```python
from build123d import *

# Parameters (mm, degrees)
BOSS_EXTRUDE1_DEPTH = 5
SKETCH2_R           = 2.55
CUT_EXTRUDE1_DEPTH  = 131.560330882
FILLET1_R           = 5


with BuildPart() as part:
    # Sketch1 → Boss-Extrude1 (new, symmetric)
    with BuildSketch(Plane.XY):
        Polygon((-49.7, 1.55), (-49.7, -11), (-5.15, -11), (-5.15, 0), (5.15, 0), (5.15, -11), (49.7, -11), (49.7, 1.55), (56, 1.55), (65, 1.55), (65, 8.55), (-65, 8.55), (-65, 1.55), (-56, 1.55), align=None)
    extrude(amount=BOSS_EXTRUDE1_DEPTH, both=True)

    # Sketch2 → Cut-Extrude1 (cut, through all)
    with BuildSketch(Plane.ZY.offset(65)):
        with Locations((0, -5.95)):
            Circle(SKETCH2_R)
    extrude(amount=-CUT_EXTRUDE1_DEPTH, mode=Mode.SUBTRACT)

    # Fillet1
    fillet1_edges = [part.edges().sort_by_distance(p)[0] for p in [
        (-27.425, -11, 5),
        (27.425, -11, 5),
        (-27.425, -11, -5),
        (27.425, -11, -5),
    ]]
    fillet(fillet1_edges, radius=FILLET1_R - 0.0001)  # a hair under: the kernel refuses the full size


solid = part.part
```
The listing builds one solid part. Answer for the finished solid, in the listing's coordinates (mm). A direction names the side the tool comes from. Coordinates: 2 decimals unless noted, no trailing zeros. Loops run counter-clockwise (first coordinate to the right, second up) from the corner with the lowest first, then second, coordinate; pieces in that order, holes last. Notation, with made-up numbers: M 8.5,-9 L 49.5,-9 A23 ccw 49.5,18 Z; hole C 19,84.5 d10. An arc over 180 degrees is marked long. Answer as a JSON object with one key per item and string values. Group by question number.
Item 1: Which of the six approach directions +Z, -Z, +X, -X, +Y, -Y give full straight-line access (tool end or side, diameter ignored) to faces 1 (the face through (-49.7, -3, 0)), 2 (the face through (57, 1.55, 0)), 3 (the face through (-5.15, -3, 0)), 4 (the face through (27.1, -8.2, 1.2)), 5 (the face through (-65, 5, 0))?
Item 2: Section A-A (y = -2) is taken. Write down the section's boundary in (x, z).
Item 3: Determine the mould class of faces 6 (the face through (0, 0, 0)), 7 (the face through (-1, 1, 5)), 8 (the face through (5.15, -3, 0)), 9 (the face through (49.7, -3, 1)) for opening direction X: +X half, -X half, draft (parallel to the pull), parting line (faces both ways), or undercut.
Item 4: Each of these flat-tipped pins is pushed along its axis until it touches: P1, Ø3, axis at x = 2, z = 0.5, coming from the -Y side; P2, Ø3, axis at y = -3, z = 2, coming from the -X side; P3, Ø3, axis at y = -6, z = 1.5, coming from the +X side. Where does it stop, or does it pass through?
Item 5: Consider L1, parallel to X at y = -3.25, z = -3; L2, parallel to Y at x = -30.5, z = 0; L3, parallel to X at y = 1, z = -4.5. Determine where each line is inside the solid, lowest interval first.
Item 6: Section C-C (x = -1.5) is taken. Write down the section's boundary in (y, z).
Solved:
{
 "1": {"face 1": "+Z, -Z, -X, -Y", "face 2": "+Z, -Z, +X, -Y", "face 3": "+Z, -Z, -Y", "face 4": "+X, -X", "face 5": "+Z, -Z, -X, +Y, -Y"},
 "2": {"outline": "M -49.7,-5 L -5.15,-5 L -5.15,5 L -49.7,5 Z; M 5.15,-5 L 49.7,-5 L 49.7,5 L 5.15,5 Z"},
 "3": {"face 6": "undercut", "face 7": "draft", "face 8": "undercut", "face 9": "+X half"},
 "4": {"P1": "stops at y = 0", "P2": "stops at x = -49.7", "P3": "stops at x = 49.7"},
 "5": {"L1": "x = -49.7 to -5.15, 5.15 to 49.7", "L2": "y = -11 to -8.5, -3.4 to 8.55", "L3": "x = -49.7 to 49.7"},
 "6": {"outline": "M 0,-5 L 8.55,-5 L 8.55,5 L 0,5 Z"}
}
